Design review of the part built by this model. Coordinates are the model's own, in mm. Face numbers are marked on the shaded views. A direction names the side the tool comes from. Round coordinates to 2 decimals unless told otherwise and drop trailing zeros. Loops run counter-clockwise (first coordinate to the right, second up) from the corner with the lowest first, then second, coordinate; pieces in that order, holes last. Notation, with made-up numbers: (73, 49) -> (113, 49) arc R35 ccw to (113, 86) -> close; hole circle Ø4 at (48, 0). An arc over 180 degrees is marked (long way). Answer as CSV lines item,"result". Start each with the question number.
(1) Take a section at D-D, the plane z = 0. State how many separate pieces and enclosed holes the cut face has, and give its area (3 significant figures).
(2) For P1, Ø7.5, axis at y = -28.575, z = 0, coming from the -X side; P2, Ø3.5, axis at y = -28.575, z = 0, coming from the -X side, all flat-tipped, find the tip position at first contact; note any pin that passes through.
(3) Take a section at B-B, the plane x = -1.75. Write out the cut boundary in (y, z) (1 decimal), and give its area (3 significant figures).
(4) To check wall thickness, follow line 1 (X direction, y = -24, z = -5) (1 decimal); line 2 (X direction, y = -27, z = -2.75) (1 decimal). State the ranges of each line that lie inside material, in increasing order. Write a range as from..to.
(5) Draft analysis for pull direction X (two halves, no side actions). For the marked faces 1, 2 and 3, state which applies: +X half, -X half, draft (parallel to the pull), parting line (faces both ways), or undercut.
(6) Take a section at A-A, the plane z = -7. Write out the cut boundary in (x, y) (1 decimal), and give its area (3 significant figures).
(7) Take a section at C-C, the plane y = -58. Write out the cut boundary in (x, z) (1 decimal).
(8) Machinability: for the marked faces 4 and 5, which of the approach directions +Z, -Z, +X, -X, +Y, -Y give a long, thin tool a straight path to every point of the face, cutting with its end or side? Answer none if there is none.
from build123d import *

# Parameters (mm, degrees)
F0_W     = 19.05
F0_H     = 19.05
F0_W_2   = 15.875
F0_H_2   = 15.875
F1_DEPTH = 76.2
F3_D     = 5.953125
F3_DEPTH = 6.35
F5_D     = 12.7
F5_DEPTH = 6.35


with BuildPart() as f1:
    # F0 (on Front) → F1 (new body)
    with BuildSketch(Plane.XZ):
        Rectangle(F0_W, F0_H)
        Rectangle(F0_W_2, F0_H_2, mode=Mode.SUBTRACT)
    extrude(amount=F1_DEPTH)

    # F3
    with Locations(Plane.YZ.offset(9.525)):
        with Locations((-9.525, 0), (-28.575, 0), (-47.625, 0)):
            Hole(F3_D / 2, depth=F3_DEPTH)

    # F5
    with Locations(Plane(origin=(-9.525, 0, 0), x_dir=(0, -1, 0), z_dir=(-1, 0, 0))):
        with Locations((9.525, 0), (28.575, 0), (47.625, 0)):
            Hole(F5_D / 2, depth=F5_DEPTH)


solid = f1.part
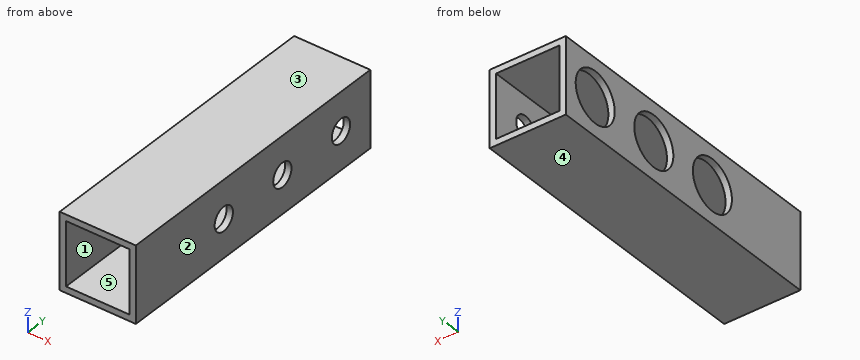
The answers:
1,separate pieces,"8"
1,enclosed holes,"0"
1,area,"153 mm²"
2,P1,"x = 7.94"
2,P2,"through"
3,outline,"(-76.2, -9.5) -> (0, -9.5) -> (0, -7.9) -> (-76.2, -7.9) -> close; (-76.2, 7.9) -> (0, 7.9) -> (0, 9.5) -> (-76.2, 9.5) -> close"
3,area,"242 mm²"
4,line 1,"-9.5..-7.9, 7.9..9.5"
4,line 2,"7.9..9.5"
5,face 1,"undercut"
5,face 2,"+X half"
5,face 3,"draft"
6,outline,"(-9.5, -76.2) -> (-7.9, -76.2) -> (-7.9, 0) -> (-9.5, 0) -> close; (7.9, -76.2) -> (9.5, -76.2) -> (9.5, 0) -> (7.9, 0) -> close"
6,area,"242 mm²"
7,outline,"(-9.5, -9.5) -> (9.5, -9.5) -> (9.5, 9.5) -> (-9.5, 9.5) -> close; hole (-7.9, -7.9) -> (7.9, -7.9) -> (7.9, 7.9) -> (-7.9, 7.9) -> close"
8,face 4,"-Z, +X, -X, +Y, -Y"
8,face 5,"+Y, -Y"
